Source: three-view drawing plus pictorial views. Frame: mm from the lowest corner of the part. A direction names the side the tool comes from. Give positions to 0.01 mm unless a question says otherwise; leave off trailing zeros. Loops run counter-clockwise (first coordinate to the right, second up) from the corner with the lowest first, then second, coordinate; pieces in that order, holes last.
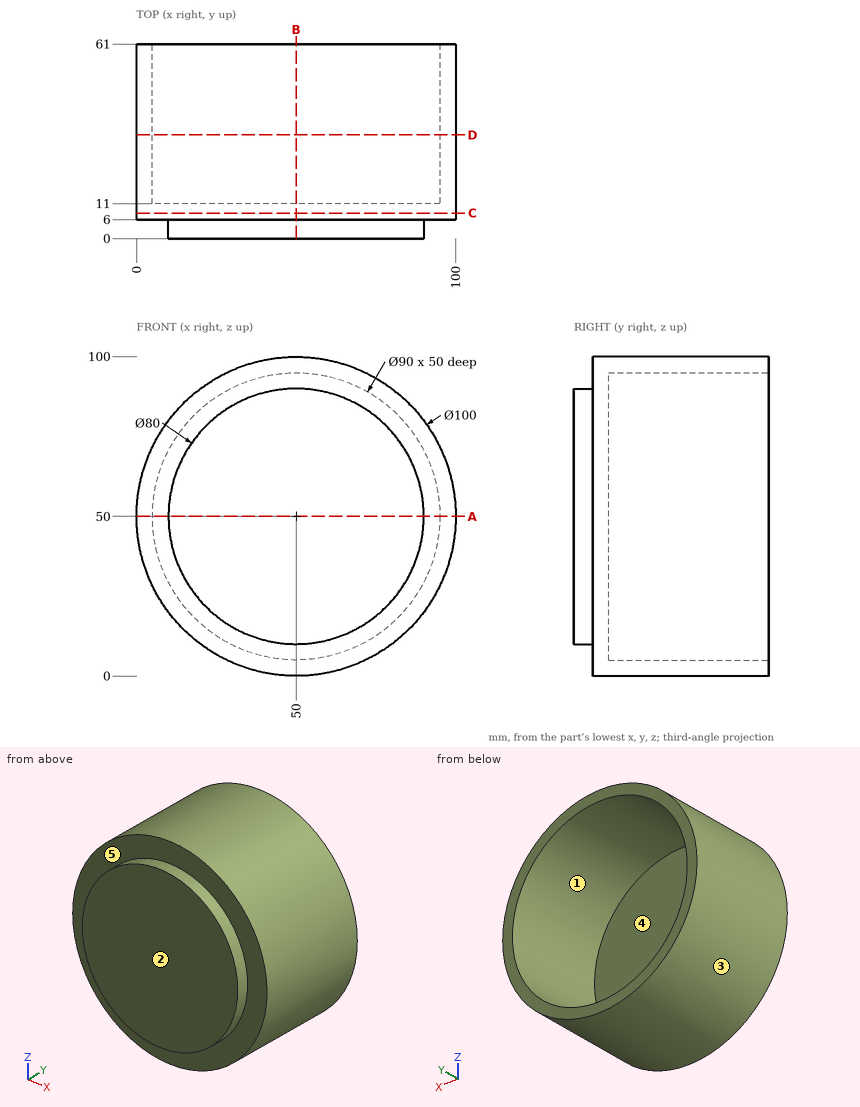
1) Reachability of the marked faces 4 and 5 from +Z, -Z, +X, -X, +Y, -Y: full face, straight path, thin tool, end or side. Return the list, or none.
Checks:
face 4: +Y
face 5: -Y
2) Cut plane D-D (y = 32.5). Return loops of the section in (x, z), and give its area (3 significant figures).
Checks:
outline: circle Ø100 at (50, 50); hole circle Ø90 at (50, 50)
area: 1,490 mm2
3) Cut plane C-C (y = 8). Return loops of the section in (x, z).
Checks:
outline: circle Ø100 at (50, 50)
4) Pull-direction query (X, two-part tool) for the marked faces 1, 2 and 3; classes: released by +X, released by -X, zero draft, split by the parting line, or undercut.
Checks:
face 1: undercut
face 2: zero draft
face 3: split by the parting line
5) Contact query for flat-ended pins moving along their axis: P1, Ø4, axis at x = 72, y = 42, coming from the -Z side; P2, Ø12, axis at x = 89, y = 8.5, coming from the -Z side; P3, Ø1.5, axis at x = 33.5, z = 77, coming from the +Y side. Output: stop coordinate, or through.
Checks:
P1: stops at z = 4.17
P2: stops at z = 12.44
P3: stops at y = 11
6) Ray query, probe 1 along Z at (x, y) = (50, 33.5); probe 2 along Y at (x, z) = (32, 18.5); probe 3 along Z at (x, y) = (59, 57). Return the intervals inside material, ascending.
Checks:
probe 1: z = 0 to 5, 95 to 100
probe 2: y = 0 to 11
probe 3: z = 0.82 to 5.91, 94.09 to 99.18
7) Cut plane A-A (z = 50). Return loops of the section in (x, y), and give its area (3 significant figures).
Checks:
outline: (0, 6) - (10, 6) - (10, 0) - (90, 0) - (90, 6) - (100, 6) - (100, 61) - (95, 61) - (95, 11) - (5, 11) - (5, 61) - (0, 61) - close
area: 1,480 mm2
8) Cut plane B-B (x = 50). Return loops of the section in (y, z).
Checks:
outline: (0, 10) - (6, 10) - (6, 0) - (61, 0) - (61, 5) - (11, 5) - (11, 95) - (61, 95) - (61, 100) - (6, 100) - (6, 90) - (0, 90) - close
